Verification items for the finished model (mm, model axes). A direction names the side the tool comes from. Round coordinates to 2 decimals unless told otherwise and drop trailing zeros. Loops run counter-clockwise (first coordinate to the right, second up) from the corner with the lowest first, then second, coordinate; pieces in that order, holes last. Notation, with made-up numbers: (-27.75, 22) - (19.25, 22) arc R19 cw to (19.25, 48) - close; hole circle Ø8 at (58, -31.75). An arc over 180 degrees is marked (long way). Use CSV: the item, a comma, the result in double quotes.
```python
from build123d import *

# Parameters (mm, degrees)
BODY_SHAFT_OUTLINE_R      = 7.75
BODY_SHAFT_DEPTH          = 14.923393759
BODY_SHAFT_START          = 14.923393759
BODY_SHAFT_2_OUTLINE_R    = 7.75
BODY_SHAFT_2_DEPTH        = 4.153212482
BODY_SHAFT_START_2        = 16.420739047
BODY_SHAFT_3_OUTLINE_W    = 18
BODY_SHAFT_3_OUTLINE_H    = 19
BODY_SHAFT_3_DEPTH        = 4.579260953
SKETCH26_W                = 6.5
SKETCH26_H                = 15.057368355
SKETCH9_R                 = 3.5
CUT_HOLE_DEPTH            = 45.218209058
CUT_SHOE_RADIUS_DEPTH     = 45.218209058
CUT_INSPECTION_HOLE_DEPTH = 45.218209058


with BuildPart() as part:
    # Body-Shaft: read off the stored shape, not the designer's step
    # Body-Shaft outline → Body-Shaft (new body)
    with BuildSketch(Plane(origin=(0, 0, 0), x_dir=(1, 0, 0), z_dir=(0, 1, 0))):
        Circle(BODY_SHAFT_OUTLINE_R)
    extrude(amount=BODY_SHAFT_DEPTH)

    # Body-Shaft 2 outline → Body-Shaft 2 (add)
    with BuildSketch(Plane(origin=(0, 0, 0), x_dir=(1, 0, 0), z_dir=(0, 1, 0)).offset(BODY_SHAFT_START)):
        Circle(BODY_SHAFT_2_OUTLINE_R)
    extrude(amount=BODY_SHAFT_2_DEPTH)

    # Body-Shaft 3 outline → Body-Shaft 3 (cut)
    with BuildSketch(Plane(origin=(0, 0, 0), x_dir=(1, 0, 0), z_dir=(0, 0.9659258262890682, 0.2588190451025211)).offset(BODY_SHAFT_START_2)):
        with Locations((0, 4.5)):
            Rectangle(BODY_SHAFT_3_OUTLINE_W, BODY_SHAFT_3_OUTLINE_H)
    extrude(amount=BODY_SHAFT_3_DEPTH, mode=Mode.SUBTRACT)

    # Sketch26 → Cut-Shaft (revolve, cut)
    with BuildSketch(Plane.XY, mode=Mode.PRIVATE) as cut_shaft_sk:
        with Locations((3.25, 7.528684178)):
            Rectangle(SKETCH26_W, SKETCH26_H)
    revolve(cut_shaft_sk.sketch.rotate(Axis((0, 0, 0), (0, 1, 0)), 270), axis=Axis((0, 0, 0), (0, 1, 0)), mode=Mode.SUBTRACT)

    # Body-Transition: read off the stored shape, not the designer's step
    # Body-Transition: loft between two sections, ruled curve by curve
    body_transition_from = [
        Edge.make_bspline([(-7.697082096, 16.75774263, 0.904116814), (-6.240942475, 13.436068349, 13.300773997), (6.240942475, 13.436068349, 13.300773997), (7.697082096, 16.75774263, 0.904116814)], [0, 0, 0, 0, 1, 1, 1, 1], 3, [1, 0.411106823, 0.411106823, 1]),
        Edge.make_bspline([(7.697082096, 16.75774263, 0.904116814), (7.767719964, 16.918878271, 0.302750415), (7.767719964, 17.081121729, -0.302750415), (7.697082096, 17.24225737, -0.904116814)], [0, 0, 0, 0, 1, 1, 1, 1], 3, [1, 0.995447922, 0.995447922, 1]),
        Edge.make_bspline([(-7.697082096, 17.24225737, -0.904116814), (-7.767719964, 17.081121729, -0.302750415), (-7.767719964, 16.918878271, 0.302750415), (-7.697082096, 16.75774263, 0.904116814)], [0, 0, 0, 0, 1, 1, 1, 1], 3, [1, 0.995447922, 0.995447922, 1]),
        Edge.make_bspline([(7.697082096, 17.24225737, -0.904116814), (6.240942475, 20.563931651, -13.300773997), (-6.240942475, 20.563931651, -13.300773997), (-7.697082096, 17.24225737, -0.904116814)], [0, 0, 0, 0, 1, 1, 1, 1], 3, [1, 0.411106823, 0.411106823, 1]),
    ]
    body_transition_to = [
        Edge.make_bspline([(-10.140902466, 24.656520189, -5.5), (-3.380300822, 24.656520189, -5.5), (3.380300822, 24.656520189, -5.5), (10.140902466, 24.656520189, -5.5)], [0, 0, 0, 0, 1, 1, 1, 1], 3),
        Edge.make_bspline([(10.140902466, 24.656520189, -5.5), (10.622491976, 23.282361026, -6.653056447), (10.622491976, 21.859541778, -7.846943553), (10.140902466, 20.485382615, -9)], [0, 0, 0, 0, 1, 1, 1, 1], 3, [1, 0.977200157, 0.977200157, 1]),
        Edge.make_bspline([(-10.140902466, 20.485382615, -9), (-10.622491976, 21.859541778, -7.846943553), (-10.622491976, 23.282361026, -6.653056447), (-10.140902466, 24.656520189, -5.5)], [0, 0, 0, 0, 1, 1, 1, 1], 3, [1, 0.977200157, 0.977200157, 1]),
        Edge.make_bspline([(10.140902466, 20.485382615, -9), (3.380300822, 20.485382615, -9), (-3.380300822, 20.485382615, -9), (-10.140902466, 20.485382615, -9)], [0, 0, 0, 0, 1, 1, 1, 1], 3),
    ]
    body_transition = Solid(Shell([*[Face.make_surface_from_curves(body_transition_from[k], body_transition_to[k]) for k in range(4)], Face(Wire(body_transition_from)), Face(Wire(body_transition_to))]))
    add(body_transition)

    # Sketch11 for Body-Shoe → Body-Shoe section 0
    with BuildSketch(Plane(origin=(0, 12.895701516, -15.368498611), x_dir=(-1, 0, 0), z_dir=(1.0474450083328146e-14, 0.6427876096865438, -0.7660444431189743))):
        with BuildLine():
            Line((10.140902466, 9.90762503), (-10.140902466, 9.90762503))
            # circular arc as an exact rational Bezier (weights 1, cos(half-angle), 1)
            Bezier((-10.140902466, 9.90762503), (-10.871813467, 12.630141727), (-10.140902466, 15.352658424), weights=[1, 0.965800235, 1])
            Line((-10.140902466, 15.352658424), (10.140902466, 15.352658424))
            Bezier((10.140902466, 15.352658424), (10.871813467, 12.630141727), (10.140902466, 9.90762503), weights=[1, 0.965800235, 1])
        make_face()
    # Sketch12 for Body-Shoe → Body-Shoe section 1
    with BuildSketch(Plane(origin=(0, 42, 0), x_dir=(-1, 0, 0), z_dir=(0, 1, 0))):
        with BuildLine():
            Line((-10.35313962, -5.5), (10.35313962, -5.5))
            Bezier((10.35313962, -5.5), (10.64894361, -7.25), (10.35313962, -9), weights=[1, 0.986013297, 1])
            Line((10.35313962, -9), (-10.35313962, -9))
            Bezier((-10.35313962, -9), (-10.64894361, -7.25), (-10.35313962, -5.5), weights=[1, 0.986013297, 1])
        make_face()
    loft()

    # Sketch9 → Cut-Hole (cut, through all)
    with BuildSketch(Plane(origin=(0, 0, 0), x_dir=(-1, 0, 0), z_dir=(0, 0, 1))):
        with Locations(Location((0, -33.328260094, 0), (0, 0, 180))):
            Circle(SKETCH9_R)
    extrude(amount=-CUT_HOLE_DEPTH, mode=Mode.SUBTRACT)

    # Sketch15 → Cut-Shoe-Radius (cut, through all)
    with BuildSketch(Plane.XY):
        with BuildLine():
            Line((10.5, 40.148566703), (10.5, 43.851433297))
            Line((10.5, 43.851433297), (-10.5, 43.851433297))
            Line((-10.5, 43.851433297), (-10.5, 40.148566703))
            ThreePointArc((-10.5, 40.148566703), (0, 42), (10.5, 40.148566703))
        make_face()
    extrude(amount=-CUT_SHOE_RADIUS_DEPTH, mode=Mode.SUBTRACT)

    # Sketch17 → Cut-Inspection-Hole (cut, through all)
    with BuildSketch(Plane.XY):
        Polygon((-1.344278322, 20.074283351), (0, 17), (1.344278322, 20.074283351), align=None)
    extrude(amount=CUT_INSPECTION_HOLE_DEPTH, mode=Mode.SUBTRACT)


solid = part.part
```
1) Thickness scan on probe 1 along X at (y, z) = (23, -7.5); probe 2 along X at (y, z) = (10.5, 0); probe 3 along Z at (x, y) = (7.75, 32.5). Record the ranges inside material, lowest first. Write a range as [from, to].
Returned:
probe 1,"x = [-10.49, 10.49]"
probe 2,"x = [-7.75, -6.5], [6.5, 7.75]"
probe 3,"z = [-9, -5.5]"
2) Cross-section at A-A, the plane y = 10. Record the cut outline in (x, z), then the cut area to 3 significant figures.
Returned:
outline,"circle Ø15.5 at (0, 0); hole circle Ø13 at (0, 0)"
area,"56.0 mm²"
3) Access from +Z, -Z, +X, -X, +Y, -Y to the whole of each face (thin tool, end or side, straight path). Record for faces 1 (the face through (0, 42, -7)), 2 (the face through (0, 15.057, 0)).
Returned:
face 1,"+Z, -Z, +Y"
face 2,"-Y"
4) Gauge pin test, flat ends, axial feed: pin 1 Ø8 at (x, y) = (1.5, 9) entering from +Z; pin 2 Ø8 at (y, z) = (9, -1) entering from +X; pin 3 Ø5 at (x, z) = (5, -3.5) entering from +Y; pin 4 Ø0.8 at (x, y) = (-0.5, 18) entering from +Z. Record the tip position at first contact, or that the pin passes through.
Returned:
pin 1,"stops at z = 7.75"
pin 2,"stops at x = 7.75"
pin 3,"stops at y = 41.8"
pin 4,"stops at z = 4.1"
5) Mould release check, pull along Z, two halves, no side actions. Record for faces 3 (the face through (-1.009, 9.405, -7.684)), 4 (the face through (-3.955, 7.634, -5.158)), 5 (the face through (0, 19, 0)): +Z half, -Z half, draft (parallel to the pull), parting line (faces both ways), or undercut.
Returned:
face 3,"parting line"
face 4,"undercut"
face 5,"+Z half"
